```python
from build123d import *

# Parameters (mm, degrees)
F0_W     = 30
F0_H     = 5.5
F1_DEPTH = 8.5
F2_SIZE  = 3
F3_SIZE2 = 1.7320508076
F3_SIZE  = 3
F5_D     = 2.5


with BuildPart() as f1:
    # F0 (on Front) → F1 (new body)
    with BuildSketch(Plane.XZ):
        Rectangle(F0_W, F0_H)
    extrude(amount=F1_DEPTH)

    # F2
    f2_edges = [f1.edges().sort_by_distance(p)[0] for p in [
        (-15, 0, 0),
        (15, 0, 0),
    ]]
    chamfer(f2_edges, length=F2_SIZE)

    # F3
    f3_edges = [f1.edges().sort_by_distance(p)[0] for p in [
        (0, -8.5, 2.75),
    ]]
    f3_side = f1.faces().sort_by_distance((0, -8.5, 0))[0]
    chamfer(f3_edges, length=F3_SIZE, length2=F3_SIZE2, reference=f3_side)

    # F5 (through all)
    with Locations(Plane.XY.offset(2.75)):
        with Locations((-10, -3), (10, -3)):
            Hole(F5_D / 2)


solid = f1.part
```
Build history of the part. All positions in model axes, mm. Give positions to 0.01 mm unless a question says otherwise; leave off trailing zeros. Loops run counter-clockwise (first coordinate to the right, second up) from the corner with the lowest first, then second, coordinate; pieces in that order, holes last. Notation, with made-up numbers: (37, 42) - (91, 42) arc R9 ccw to (91, 48) - close; hole circle Ø11 at (71, 30). An arc over 180 degrees is marked (long way). Use a Markdown table: item, result.
(1) Band-saw the part on B-B (x = -10). Give the cut face in (y, z).
Taken from the geometry:
| item | result |
|---|---|
| outline | (-8.5, -2.75) - (-4.25, -2.75) - (-4.25, 2.75) - (-6.77, 2.75) - (-8.5, -0.25) - close; (-1.75, -2.75) - (0, -2.75) - (0, 2.75) - (-1.75, 2.75) - close |
(2) Band-saw the part on C-C (z = 1.65). Give the cut face in (x, y), and give its area (3 significant figures).
Taken from the geometry:
| item | result |
|---|---|
| outline | (-15, -7.4) - (15, -7.4) - (15, -3) - (12, 0) - (-12, 0) - (-15, -3) - close; hole circle Ø2.5 at (-10, -3); hole circle Ø2.5 at (10, -3) |
| area | 203 mm2 |
(3) Band-saw the part on D-D (x = 13.25). Give the cut face in (y, z), and give its area (3 significant figures).
Taken from the geometry:
| item | result |
|---|---|
| outline | (-8.5, -2.75) - (-1.25, -2.75) - (-1.25, 2.75) - (-6.77, 2.75) - (-8.5, -0.25) - close |
| area | 37.3 mm2 |
(4) Pull direction X, two halves, no side cores. Call faces 1 (the face through (-8.75, -2.95, -0.04)), 2 (the face through (0, -3, 2.75)), 3 (the face through (-13, -1, 0)): +X half, -X half, draft (parallel to the pull), parting line (faces both ways), or undercut.
Taken from the geometry:
| item | result |
|---|---|
| face 1 | undercut |
| face 2 | draft |
| face 3 | -X half |
(5) Band-saw the part on A-A (y = -2.25). Give the cut face in (x, z), and give its area (3 significant figures).
Taken from the geometry:
| item | result |
|---|---|
| outline | (-14.25, -2.75) - (-11, -2.75) - (-11, 2.75) - (-14.25, 2.75) - close; (-9, -2.75) - (9, -2.75) - (9, 2.75) - (-9, 2.75) - close; (11, -2.75) - (14.25, -2.75) - (14.25, 2.75) - (11, 2.75) - close |
| area | 135 mm2 |
(6) Wall check: line 1 along X through (y, z) = (-2.5, -2.25); line 2 along Y through (x, z) = (-10, -0.3); line 3 along X through (y, z) = (-2.75, -0.65). Give the ranges that are in metal, low to high.
Taken from the geometry:
| item | result |
|---|---|
| line 1 | -14.5 to -11.15, -8.85 to 8.85, 11.15 to 14.5 |
| line 2 | -8.5 to -4.25, -1.75 to 0 |
| line 3 | -14.75 to -11.22, -8.78 to 8.78, 11.22 to 14.75 |
(7) Drop a flat-ended pin along its axis: pin 1 Ø2 at (x, y) = (10, -3) entering from -Z (3 decimals). Give the stop position or say it passes through.
Taken from the geometry:
| item | result |
|---|---|
| pin 1 | through |
